Work out the finished part from the listing and answer in its coordinate system (mm). Face numbers are marked on the shaded views. A direction names the side the tool comes from. Coordinates: 2 decimals unless noted, no trailing zeros. Order: outer loops, then holes, each group sorted by start corner. A loop starts at its lowest first (then second) coordinate and runs counter-clockwise, first axis right, second up. Notation, with made-up numbers: (0.25, 77) - (45.25, 77) arc R33 cw to (45.25, 105) - close; hole circle Ø9 at (39.5, 31). An arc over 180 degrees is marked (long way). Answer as a JSON object with one key per item and string values. Group by question number.
1) Section C-C (x = 0) is taken. Count the separate pieces of the cut face and the enclosed holes in it, plus the area to 3 significant figures.
2) Section B-B (z = 7.25) is taken. Give the vertices of the cut face in (x, y).
3) Each of these flat-tipped pins is pushed along its axis until it touches: P1, Ø2.5, axis at x = -20.78, y = 45.5, coming from the +Z side; P2, Ø4, axis at x = -23.5, y = -61, coming from the -Z side (3 decimals); P3, Ø6, axis at x = 6, z = 5.5, coming from the +Y side; P4, Ø4, axis at y = -10, z = 16.5, coming from the -X side. Where does it stop, or does it pass through?
4) Find the intervals of material crossed by line 1 along X through (y, z) = (-4.5, 9.25); line 2 along Y through (x, z) = (-3, 17.5); line 3 along Y through (x, z) = (-18, 9), in increasing order.
5) A tool of negligible diameter and unlimited length cuts with its end or side. For the marked faces 1, 2, 3 and 4, from which of +Z, -Z, +X, -X, +Y, -Y can it reach the whole face along a straight path? Write none if from no direction.
6) The mould has two halves that part along X. Classify the marked faces 5, 6 and 7: released by +X, released by -X, zero draft, split by the parting line, or undercut.
7) Section A-A (y = 42) is taken. Give the vertices of the cut face in (x, z) (3 decimals), plus the area to 3 significant figures.
from build123d import *
from build123d.topology import SkipClean

# Parameters (mm, degrees)
SKETCH1_R           = 27.5
BOSS_EXTRUDE1_DEPTH = 20
BOSS_EXTRUDE2_START = -3.175
SKETCH2_R           = 20
SKETCH2_R_2         = 2
BOSS_EXTRUDE2_DEPTH = 3.175
CUT_EXTRUDE6_DEPTH  = 44
FILLET4_R           = 5
SKETCH9_R           = 27.302550199
SKETCH9_R_2         = 27.201682831
BOSS_EXTRUDE3_DEPTH = 12.5
SKETCH12_W          = 50.8
SKETCH12_H          = 50.8
CUT_EXTRUDE7_DEPTH  = 12.5


with BuildPart() as part:
    # Sketch1 → Boss-Extrude1 (new body)
    with BuildSketch(Plane.XY):
        with BuildLine():
            Line((-29.75, 57.5), (-29.75, -57.5))
            ThreePointArc((-29.75, -57.5), (0, -87.25), (29.75, -57.5))
            Line((29.75, -57.5), (29.75, 57.5))
            ThreePointArc((29.75, 57.5), (0, 87.25), (-29.75, 57.5))
        make_face()
        with Locations((0, 57.5)):
            Circle(SKETCH1_R, mode=Mode.SUBTRACT)
        with Locations(Location((0, -57.5, 0), (0, 0, 180))):
            Circle(SKETCH1_R, mode=Mode.SUBTRACT)
    extrude(amount=BOSS_EXTRUDE1_DEPTH)

    # Sketch2 → Boss-Extrude2 (add)
    with BuildSketch(Plane.XY.offset(20).offset(BOSS_EXTRUDE2_START)):
        with BuildLine():
            Line((-29.75, 57.5), (-29.75, -57.5))
            ThreePointArc((-29.75, -57.5), (0, -87.25), (29.75, -57.5))
            Line((29.75, -57.5), (29.75, 57.5))
            ThreePointArc((29.75, 57.5), (0, 87.25), (-29.75, 57.5))
        make_face()
        with Locations((0, 57.5)):
            Circle(SKETCH2_R, mode=Mode.SUBTRACT)
        with Locations((0, 81.5)):
            Circle(SKETCH2_R_2, mode=Mode.SUBTRACT)
        with Locations((20.784609691, 69.5)):
            Circle(SKETCH2_R_2, mode=Mode.SUBTRACT)
        with Locations((20.784609691, 45.5)):
            Circle(SKETCH2_R_2, mode=Mode.SUBTRACT)
        with Locations((0, 33.5)):
            Circle(SKETCH2_R_2, mode=Mode.SUBTRACT)
        with Locations((-20.784609691, 45.5)):
            Circle(SKETCH2_R_2, mode=Mode.SUBTRACT)
        with Locations((-20.784609691, 69.5)):
            Circle(SKETCH2_R_2, mode=Mode.SUBTRACT)
        with Locations(Location((-20.784609691, -69.5, 0), (0, 0, 180))):
            Circle(SKETCH2_R_2, mode=Mode.SUBTRACT)
        with Locations(Location((-20.784609691, -45.5, 0), (0, 0, 180))):
            Circle(SKETCH2_R_2, mode=Mode.SUBTRACT)
        with Locations(Location((0, -33.5, 0), (0, 0, 180))):
            Circle(SKETCH2_R_2, mode=Mode.SUBTRACT)
        with Locations(Location((20.784609691, -45.5, 0), (0, 0, 180))):
            Circle(SKETCH2_R_2, mode=Mode.SUBTRACT)
        with Locations(Location((20.784609691, -69.5, 0), (0, 0, 180))):
            Circle(SKETCH2_R_2, mode=Mode.SUBTRACT)
        with Locations(Location((0, -81.5, 0), (0, 0, 180))):
            Circle(SKETCH2_R_2, mode=Mode.SUBTRACT)
        with Locations(Location((0, -57.5, 0), (0, 0, 180))):
            Circle(SKETCH2_R, mode=Mode.SUBTRACT)
    extrude(amount=BOSS_EXTRUDE2_DEPTH)

    # Sketch8 → Cut-Extrude6 (cut)
    with SkipClean():  # the faces are left unmerged after this step: merging them gives an invalid solid
        with BuildSketch(Plane(origin=(0, 0, 0), x_dir=(-1, 0, 0), z_dir=(0, 0, -1))):
            with BuildLine():
                Line((-2.5, -27.855228117), (-2.5, 27.855228117))
                ThreePointArc((-2.5, 27.855228117), (-21.902482736, 37.366849477), (-29.75, 57.5))
                Line((-29.75, 57.5), (-29.75, -57.5))
                ThreePointArc((-29.75, -57.5), (-21.902482736, -37.366849477), (-2.5, -27.855228117))
            make_face()
            with BuildLine():
                Line((2.5, -27.855228117), (2.5, 27.855228117))
                ThreePointArc((2.5, 27.855228117), (21.902482736, 37.366849477), (29.75, 57.5))
                Line((29.75, 57.5), (29.75, -57.5))
                ThreePointArc((29.75, -57.5), (21.902482736, -37.366849477), (2.5, -27.855228117))
            make_face()
        extrude(amount=-CUT_EXTRUDE6_DEPTH, mode=Mode.SUBTRACT)

    # Fillet4
    fillet4_edges = [part.edges().sort_by_distance(p)[0] for p in [
        (2.5, -27.855228117, 10),
        (2.5, 27.855228117, 10),
        (-2.5, 27.855228117, 10),
        (-2.5, -27.855228117, 10),
    ]]
    fillet(fillet4_edges, radius=FILLET4_R)

    # Sketch9 → Boss-Extrude3 (add)
    with BuildSketch(Plane.XY):
        with BuildLine():
            Line((-29.75, 57.5), (-29.75, -57.5))
            ThreePointArc((-29.75, -57.5), (0, -87.25), (29.75, -57.5))
            Line((29.75, -57.5), (29.75, 57.5))
            ThreePointArc((29.75, 57.5), (0, 87.25), (-29.75, 57.5))
        make_face()
        with Locations((0, 57.5)):
            Circle(SKETCH9_R, mode=Mode.SUBTRACT)
        with Locations((0, -57.5)):
            Circle(SKETCH9_R_2, mode=Mode.SUBTRACT)
    extrude(amount=BOSS_EXTRUDE3_DEPTH)

    # Sketch12 → Cut-Extrude7 (cut)
    with BuildSketch(Plane(origin=(0, 0, 0), x_dir=(-1, 0, 0), z_dir=(0, 0, -1))):
        Rectangle(SKETCH12_W, SKETCH12_H)
    extrude(amount=-CUT_EXTRUDE7_DEPTH, mode=Mode.SUBTRACT)


solid = part.part
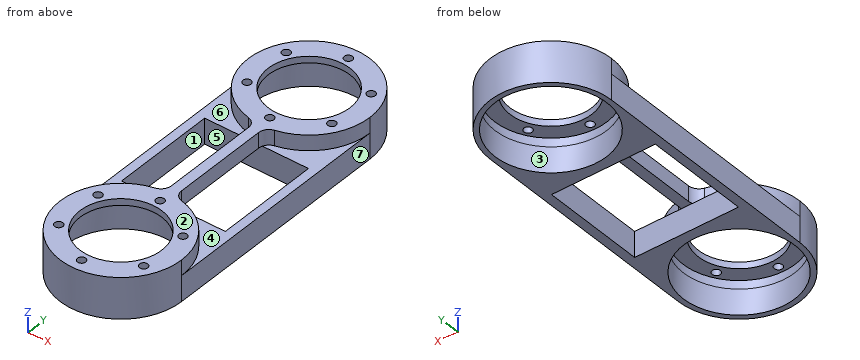
Report:
{
 "1": {"separate pieces": "7", "enclosed holes": "0", "area": "712 mm²"},
 "2": {"outline": "(-29.75, -57.5) arc R29.75 ccw to (29.75, -57.5) - (29.75, 57.5) arc R29.75 ccw to (-29.75, 57.5) - close; hole circle Ø54.61 at (0, 57.5); hole circle Ø54.4 at (0, -57.5); hole (-25.4, -25.4) - (25.4, -25.4) - (25.4, 25.4) - (-25.4, 25.4) - close"},
 "3": {"P1": "passes through", "P2": "stops at z = 16.825", "P3": "stops at y = 87.1", "P4": "stops at x = -2.5"},
 "4": {"line 1": "x = -29.75 to -25.4, 25.4 to 29.75", "line 2": "y = -87.1 to -77.27, -37.73 to -25.75, 25.75 to 37.73, 77.27 to 87.1", "line 3": "y = -81.19 to -77.89, -37.11 to -25.4, 25.4 to 36.97, 78.03 to 81.19"},
 "5": {"face 1": "+Z, -Z", "face 2": "+Z, +X, -X, +Y, -Y", "face 3": "-Z", "face 4": "+Z, +X"},
 "6": {"face 5": "undercut", "face 6": "zero draft", "face 7": "released by +X"},
 "7": {"outline": "(-29.75, 0) - (-22.476, 0) - (-22.476, 12.5) - (-22.716, 12.5) - (-22.716, 16.825) - (-12.639, 16.825) - (-12.639, 20) - (-25.393, 20) - (-25.393, 12.5) - (-29.75, 12.5) - close; (12.639, 16.825) - (22.716, 16.825) - (22.716, 12.5) - (22.476, 12.5) - (22.476, 0) - (29.75, 0) - (29.75, 12.5) - (25.393, 12.5) - (25.393, 20) - (12.639, 20) - close", "area": "286 mm²"}
}
